from build123d import *

# Parameters (mm, degrees)
SKETCH_2_R               = 10.75
SKETCH_2_R_2             = 0.5
EXTRUDE_1_DEPTH          = 2
EXTRUDE_3_DEPTH          = 2
SKETCH_4_W               = 2
SKETCH_4_H               = 33
EXTRUDE_4_DEPTH          = 75
SKETCH_8_R               = 0.7
CUT_EXTRUDE_1_DEPTH      = 7
SKETCH_9_W               = 2
SKETCH_9_H               = 21.5
EXTRUDE_7_DEPTH          = 60
EXTRUDE_2_DEPTH          = 2
SKETCH_11_R              = 2.4
EXTRUDE_8_DEPTH          = 15
SKETCH_12_W              = 59
SKETCH_12_H              = 30
CUT_EXTRUDE_2_DEPTH      = 15
SKETCH_13_W              = 59
SKETCH_13_H              = 1.5
EXTRUDE_9_DEPTH          = 4.5
SKETCH_15_W              = 6.749564512
SKETCH_15_H              = 21.5
EXTRUDE_10_DEPTH         = 2
SKETCH_16_W              = 6.749564512
SKETCH_16_H              = 21.5
EXTRUDE_11_DEPTH         = 2
CUT_EXTRUDE_3_DEPTH      = 173.33717765
CUT_EXTRUDE_3_DEPTH_BACK = 173.33717765
SKETCH_17_R              = 1.5


with BuildPart() as part:
    # 스케치2 → 보스-돌출1 (new body)
    with BuildSketch(Plane(origin=(62.38287134, 0, 0), x_dir=(0, 0, -1), z_dir=(1, 0, 0))):
        with Locations((-65.677419436, 69.66810471)):
            Circle(SKETCH_2_R)
        with Locations((-61.803243354, 76.447725619)):
            Circle(SKETCH_2_R_2, mode=Mode.SUBTRACT)
        with Locations((-65.040124528, 76.73944512)):
            Circle(SKETCH_2_R_2, mode=Mode.SUBTRACT)
        with Locations((-68.277005701, 77.03116462)):
            Circle(SKETCH_2_R_2, mode=Mode.SUBTRACT)
        with Locations((-72.457040346, 73.542280792)):
            Circle(SKETCH_2_R_2, mode=Mode.SUBTRACT)
        with Locations((-72.748759847, 70.305399618)):
            Circle(SKETCH_2_R_2, mode=Mode.SUBTRACT)
        with Locations((-73.040479347, 67.068518444)):
            Circle(SKETCH_2_R_2, mode=Mode.SUBTRACT)
        with Locations((-69.551595519, 62.8884838)):
            Circle(SKETCH_2_R_2, mode=Mode.SUBTRACT)
        with Locations((-66.314714345, 62.596764299)):
            Circle(SKETCH_2_R_2, mode=Mode.SUBTRACT)
        with Locations((-63.077833171, 62.305044799)):
            Circle(SKETCH_2_R_2, mode=Mode.SUBTRACT)
        with Locations((-58.897798526, 65.793928627)):
            Circle(SKETCH_2_R_2, mode=Mode.SUBTRACT)
        with Locations((-58.606079026, 69.030809801)):
            Circle(SKETCH_2_R_2, mode=Mode.SUBTRACT)
        with Locations((-58.314359525, 72.267690975)):
            Circle(SKETCH_2_R_2, mode=Mode.SUBTRACT)
    extrude(amount=EXTRUDE_1_DEPTH)

    # 스케치3 → 보스-돌출3 (add)
    with BuildSketch(Plane.ZY.offset(-62.38287134)):
        with BuildLine():
            Line((65.677419436, 80.41810471), (127.677419436, 80.41810471))
            Line((127.677419436, 80.41810471), (127.677419436, 58.91810471))
            Line((127.677419436, 58.91810471), (65.677419436, 58.91810471))
            ThreePointArc((65.677419436, 58.91810471), (76.427419436, 69.66810471), (65.677419436, 80.41810471))
        make_face()
    extrude(amount=-EXTRUDE_3_DEPTH)

    # 스케치4 → 보스-돌출4 (add)
    with BuildSketch(Plane.ZY.offset(-62.38287134)):
        with Locations((126.677419436, 69.66810471)):
            Rectangle(SKETCH_4_W, SKETCH_4_H)
    extrude(amount=EXTRUDE_4_DEPTH)

    # 스케치8 → 컷-돌출1 (cut)
    with BuildSketch(Plane(origin=(64.38287134, 0, 0), x_dir=(0, 0, -1), z_dir=(1, 0, 0))):
        with Locations((-68.277005701, 77.03116462)):
            Circle(SKETCH_8_R)
        with Locations((-65.040124528, 76.73944512)):
            Circle(SKETCH_8_R)
        with Locations((-61.803243354, 76.447725619)):
            Circle(SKETCH_8_R)
        with Locations((-58.314359525, 72.267690975)):
            Circle(SKETCH_8_R)
        with Locations((-58.606079026, 69.030809801)):
            Circle(SKETCH_8_R)
        with Locations((-58.897798526, 65.793928627)):
            Circle(SKETCH_8_R)
        with Locations((-63.077833171, 62.305044799)):
            Circle(SKETCH_8_R)
        with Locations((-66.314714345, 62.596764299)):
            Circle(SKETCH_8_R)
        with Locations((-69.551595519, 62.8884838)):
            Circle(SKETCH_8_R)
        with Locations((-73.040479347, 67.068518444)):
            Circle(SKETCH_8_R)
        with Locations((-72.748759847, 70.305399618)):
            Circle(SKETCH_8_R)
        with Locations((-72.457040346, 73.542280792)):
            Circle(SKETCH_8_R)
    extrude(amount=-CUT_EXTRUDE_1_DEPTH, mode=Mode.SUBTRACT)

    # 스케치9 → 보스-돌출7 (add)
    with BuildSketch(Plane(origin=(0, 0, 125.677419436), x_dir=(-1, 0, 0), z_dir=(0, 0, -1))):
        with Locations((11.61712866, 69.66810471)):
            Rectangle(SKETCH_9_W, SKETCH_9_H)
    extrude(amount=EXTRUDE_7_DEPTH)

    # 스케치10 → 돌출-얇게2 (add)
    with BuildSketch(Plane.ZY.offset(12.61712866)):
        with BuildLine():
            ThreePointArc((65.677419436, 80.41810471), (54.927419436, 69.66810471), (65.677419436, 58.91810471))
            Line((65.677419436, 58.91810471), (65.677419436, 68.91810471))
            ThreePointArc((65.677419436, 68.91810471), (64.927419436, 69.66810471), (65.677419436, 70.41810471))
            Line((65.677419436, 70.41810471), (65.677419436, 80.41810471))
        make_face()
    extrude(amount=-EXTRUDE_2_DEPTH)

    # 스케치11 → 보스-돌출8 (add)
    with BuildSketch(Plane.ZY.offset(12.61712866)):
        with Locations((65.677419436, 69.66810471)):
            Circle(SKETCH_11_R)
    extrude(amount=-EXTRUDE_8_DEPTH)

    # 스케치12 → 컷-돌출2 (cut)
    with BuildSketch(Plane.XY.offset(127.677419436)):
        with Locations((24.88287134, 69.66810471)):
            Rectangle(SKETCH_12_W, SKETCH_12_H)
    extrude(amount=-CUT_EXTRUDE_2_DEPTH, mode=Mode.SUBTRACT)

    # 스케치13 → 보스-돌출9 (add, symmetric)
    with BuildSketch(Plane(origin=(0, 0, 125.677419436), x_dir=(-1, 0, 0), z_dir=(0, 0, -1))):
        with Locations((-24.88287134, 53.91810471)):
            Rectangle(SKETCH_13_W, SKETCH_13_H)
        with Locations((-24.88287134, 85.41810471)):
            Rectangle(SKETCH_13_W, SKETCH_13_H)
    extrude(amount=EXTRUDE_9_DEPTH, both=True)

    # 스케치15 → 보스-돌출10 (add)
    with BuildSketch(Plane.ZY.offset(-62.38287134)):
        with Locations((122.30263718, 69.66810471)):
            Rectangle(SKETCH_15_W, SKETCH_15_H)
    extrude(amount=EXTRUDE_10_DEPTH)

    # 스케치16 → 보스-돌출11 (add)
    with BuildSketch(Plane(origin=(-10.61712866, 0, 0), x_dir=(0, 0, -1), z_dir=(1, 0, 0))):
        with Locations((-122.30263718, 69.66810471)):
            Rectangle(SKETCH_16_W, SKETCH_16_H)
    extrude(amount=EXTRUDE_11_DEPTH)

    # 스케치17 → 컷-돌출3 (cut, two sides: drawn at the far end of the back side and taken through both)
    with BuildSketch(Plane.ZY.offset(-60.38287134).offset(-CUT_EXTRUDE_3_DEPTH_BACK)):
        with Locations((122.30263718, 74.43740033)):
            Circle(SKETCH_17_R)
        with Locations((122.30263718, 64.421879527)):
            Circle(SKETCH_17_R)
    extrude(amount=CUT_EXTRUDE_3_DEPTH + CUT_EXTRUDE_3_DEPTH_BACK, mode=Mode.SUBTRACT)


solid = part.part
The model under review builds one solid part; all positions refer to its coordinate system, in mm. A direction names the side the tool comes from. Give positions to 0.01 mm unless a question says otherwise; leave off trailing zeros. Order: outer loops, then holes, each group sorted by start corner. A loop starts at its lowest first (then second) coordinate and runs counter-clockwise, first axis right, second up. Notation, with made-up numbers: M -36,68.25 L 22,68.25 A7 ccw 22,76.25 Z; hole C 27.25,6 d5. An arc over 180 degrees is marked long. Answer in a Markdown table with one row per item. Add a question column.
1. Mouldability with a two-part tool opening along Y and no side actions: class faces 4 (the flat face through (64.383, 70, 92)), 5 (the flat face through (-11, 80.418, 96)), 6 (the cylindrical face through (-10.589, 75.451, 121.197)) as released by +Y, released by -Y, zero draft, split by the parting line, or undercut.
2. Add section D-D on x = -7. State the section outline as (y, z) points, plus the area to 3 significant figures.
3. Add section B-B on z = 103.5. State the section outline as (x, y) points, plus the area to 3 significant figures.
4. For pin 1 Ø1.8 at (y, z) = (74.44, 122.3) entering from +X; pin 2 Ø1.2 at (y, z) = (53.5, 129) entering from -X; pin 3 Ø1.2 at (x, y) = (31, 85.5) entering from -Z; pin 4 Ø2 at (x, z) = (-11.5, 102) entering from +Y, all flat-tipped, find the tip position at first contact; note any pin that passes through.
5. Add section C-C on x = 55.5. State the section outline as (y, z) points, plus the area to 3 significant figures.
6. To check wall thickness, follow line 1 along Y through (x, z) = (41, 126); line 2 along X through (y, z) = (77.5, 94); line 3 along X through (y, z) = (59.5, 122). State the ranges of each line that lie inside material, in increasing order.
7. Machinability: for faces 1 (the cylindrical face through (-4.21, 69.77, 63.28)), 2 (the flat face through (24, 54.668, 126)), 3 (the flat face through (60.383, 70, 122)), which of the approach directions +Z, -Z, +X, -X, +Y, -Y give a long, thin tool a straight path to every point of the face, cutting with its end or side? Answer none if there is none.
8. Add section A-A on x = 12. State the section outline as (y, z) points, plus the area to 3 significant figures.
The answers:
| question | item | result |
|---|---|---|
| 1 | face 4 | zero draft |
| 1 | face 5 | released by +Y |
| 1 | face 6 | undercut |
| 2 | outline | M 53.17,125.68 L 86.17,125.68 L 86.17,127.68 L 53.17,127.68 Z; C 69.67,65.68 d4.8 |
| 2 | area | 84.1 mm2 |
| 3 | outline | M -12.62,58.92 L -10.62,58.92 L -10.62,80.42 L -12.62,80.42 Z; M 62.38,58.92 L 64.38,58.92 L 64.38,80.42 L 62.38,80.42 Z |
| 3 | area | 86.0 mm2 |
| 4 | pin 1 | through |
| 4 | pin 2 | x = -4.62 |
| 4 | pin 3 | z = 121.18 |
| 4 | pin 4 | y = 80.42 |
| 5 | outline | M 53.17,125.68 L 86.17,125.68 L 86.17,127.68 L 53.17,127.68 Z |
| 5 | area | 66.0 mm2 |
| 6 | line 1 | 53.17 to 54.67, 84.67 to 86.17 |
| 6 | line 2 | -12.62 to -10.62, 62.38 to 64.38 |
| 6 | line 3 | -12.62 to -8.62, 60.38 to 64.38 |
| 7 | face 1 | none |
| 7 | face 2 | +Z, -Z |
| 7 | face 3 | -Z, +Y, -Y |
| 8 | outline | M 53.17,121.18 L 54.67,121.18 L 54.67,130.18 L 53.17,130.18 Z; M 84.67,121.18 L 86.17,121.18 L 86.17,130.18 L 84.67,130.18 Z |
| 8 | area | 27.0 mm2 |
